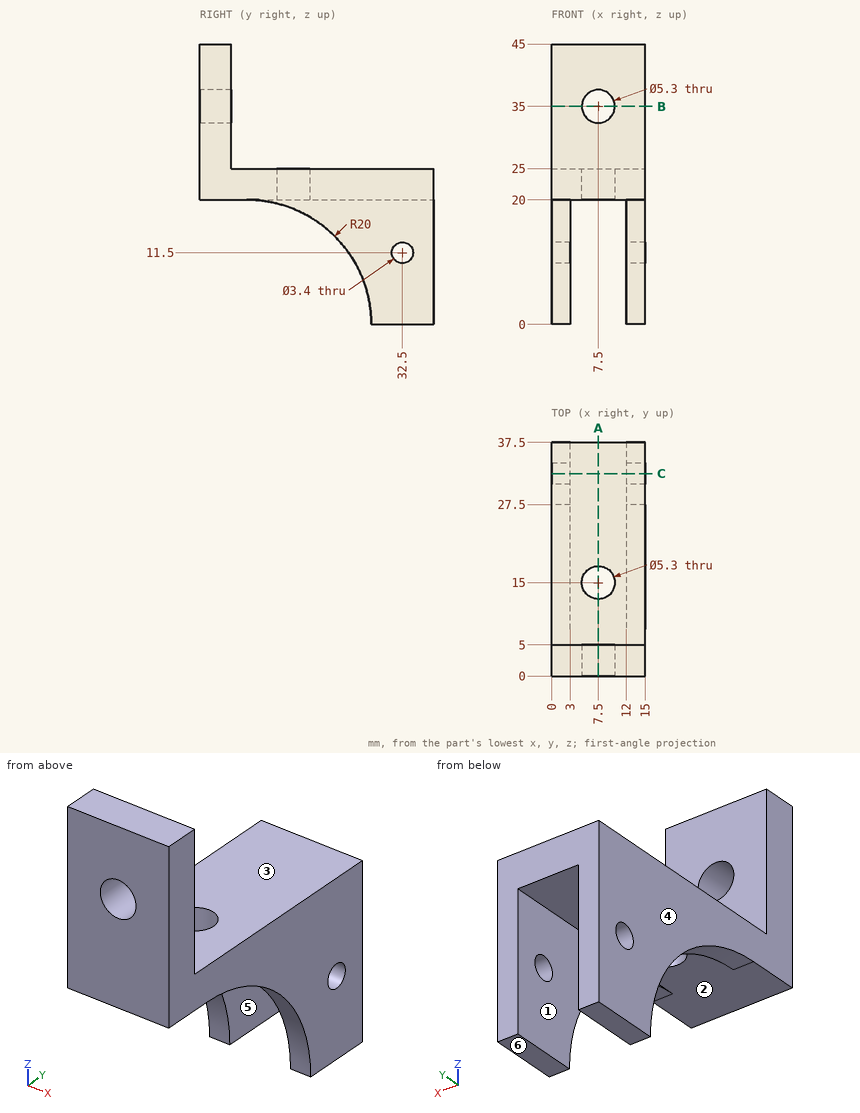
Geometry check sheet. Reference: drawing and pictorial views, mm from the part's lowest x, y, z. A direction names the side the tool comes from. Give positions to 0.01 mm unless a question says otherwise; leave off trailing zeros. Loops run counter-clockwise (first coordinate to the right, second up) from the corner with the lowest first, then second, coordinate; pieces in that order, holes last. Notation, with made-up numbers: (24.5, 23.5) -> (37.5, 23.5) arc R8 cw to (37.5, 36.5) -> close; hole circle Ø8 at (-31.5, 74). An arc over 180 degrees is marked (long way). Answer in a Markdown table with one row per item. Add a question column.
1) Material ranges on probe 1 along Y at (x, z) = (7.5, 21.7); probe 2 along Z at (x, y) = (2.25, 32.5); probe 3 along X at (y, z) = (34.5, 17), recorded low to high. Write a range as from..to.
2) Cross-section at C-C on y = 32.5. Record the boundary of the cut face in (x, z), and give its area (3 significant figures).
3) Set-up check for the marked faces 1, 2 and 3: record each of +Z, -Z, +X, -X, +Y, -Y from which the full face is reachable in a straight line by a thin tool's end or side.
4) Cross-section at B-B on z = 35. Record the boundary of the cut face in (x, y), and give its area (3 significant figures).
5) Gauge pin test, flat ends, axial feed: P1, Ø4.5, axis at x = 7.5, y = 15.5, coming from the -Z side; P2, Ø22, axis at y = 16, z = 15, coming from the -X side; P3, Ø7.5, axis at x = 4, y = 13.5, coming from the +Z side; P4, Ø7.5, axis at x = 8.5, z = 37, coming from the +Y side. Record the tip position at first contact, or that the pin passes through.
6) Draft check along X on the marked faces 4, 5 and 6. Enter one of: pulls with the +X half, pulls with the -X half, needs draft (parallel to the pull), parting line crosses it, or undercut.
7) Cross-section at A-A on x = 7.5. Record the boundary of the cut face in (y, z), and give its area (4 significant figures).
Outcome:
| question | item | result |
|---|---|---|
| 1 | probe 1 | y = 0..12.35, 17.65..37.5 |
| 1 | probe 2 | z = 0..9.8, 13.2..25 |
| 1 | probe 3 | x = 0..3, 12..15 |
| 2 | outline | (0, 0) -> (3, 0) -> (3, 9.8) -> (0, 9.8) -> close; (0, 13.2) -> (3, 13.2) -> (3, 20) -> (12, 20) -> (12, 13.2) -> (15, 13.2) -> (15, 25) -> (0, 25) -> close; (12, 0) -> (15, 0) -> (15, 9.8) -> (12, 9.8) -> close |
| 2 | area | 175 mm^2 |
| 3 | face 1 | -Z, +Y, -Y |
| 3 | face 2 | -Z, -Y |
| 3 | face 3 | +Z, +X, -X, +Y |
| 4 | outline | (0, 0) -> (4.85, 0) -> (4.85, 5) -> (0, 5) -> close; (10.15, 0) -> (15, 0) -> (15, 5) -> (10.15, 5) -> close |
| 4 | area | 48.5 mm^2 |
| 5 | P1 | stops at z = 20 |
| 5 | P2 | stops at x = 0 |
| 5 | P3 | stops at z = 25 |
| 5 | P4 | stops at y = 5 |
| 6 | face 4 | pulls with the -X half |
| 6 | face 5 | undercut |
| 6 | face 6 | needs draft |
| 7 | outline | (0, 20) -> (12.35, 20) -> (12.35, 25) -> (5, 25) -> (5, 32.35) -> (0, 32.35) -> close; (0, 37.65) -> (5, 37.65) -> (5, 45) -> (0, 45) -> close; (17.65, 20) -> (37.5, 20) -> (37.5, 25) -> (17.65, 25) -> close |
| 7 | area | 234.5 mm^2 |
